```python
from build123d import *

# Parameters (mm, degrees)
SKETCH_R        = 16
PAD_DEPTH       = 35
SKETCH001_R     = 14
POCKET_DEPTH    = 23
SKETCH002_R     = 3.98
PAD001_DEPTH    = 10
SKETCH003_W     = 5.2
SKETCH003_H     = 1.2
POCKET001_DEPTH = 10
SKETCH004_W     = 4.2
SKETCH004_H     = 32.681076
POCKET002_DEPTH = 10


with BuildPart() as part:
    # Sketch → Pad (new body)
    with BuildSketch(Plane.XY):
        Circle(SKETCH_R)
    extrude(amount=PAD_DEPTH)

    # Sketch001 (on Face2 of Pad) → Pocket (cut)
    with BuildSketch(Plane(origin=(0, 0, 0), x_dir=(1, 0, 0), z_dir=(0, 0, -1))):
        Circle(SKETCH001_R)
    extrude(amount=-POCKET_DEPTH, mode=Mode.SUBTRACT)

    # Sketch002 (on Face5 of Pocket) → Pad001 (join)
    with BuildSketch(Plane(origin=(0, 0, 23), x_dir=(1, 0, 0), z_dir=(0, 0, -1))):
        Circle(SKETCH002_R)
    extrude(amount=PAD001_DEPTH)

    # Sketch003 (on Face3 of Pad001) → Pocket001 (cut)
    with BuildSketch(Plane.XY.offset(35)):
        Rectangle(SKETCH003_W, SKETCH003_H)
    extrude(amount=-POCKET001_DEPTH, mode=Mode.SUBTRACT)

    # Sketch004 (on Face3 of Pocket001) → Pocket002 (cut)
    with BuildSketch(Plane.XY.offset(35)):
        with Locations((0, -0.015375)):
            Rectangle(SKETCH004_W, SKETCH004_H)
    extrude(amount=-POCKET002_DEPTH, mode=Mode.SUBTRACT)


solid = part.part
```
Source: CAD feature listing. Evaluate the final solid. Frame: model axes, mm. A direction names the side the tool comes from. Round coordinates to 2 decimals unless told otherwise and drop trailing zeros. Loops run counter-clockwise (first coordinate to the right, second up) from the corner with the lowest first, then second, coordinate; pieces in that order, holes last. Notation, with made-up numbers: M -30,3 L 15,3 A33 cw 15,33 Z; hole C 13,43.5 d6. An arc over 180 degrees is marked long. Use a Markdown table: item, result. Add a question column.
1. Pull-direction query (X, two-part tool) for faces 1 (the flat face through (-8, 0, 35)), 2 (the flat face through (2.6, 0, 30)), 3 (the cylindrical face through (-3.47, -15.62, 17.26)), 4 (the cylindrical face through (12.932, 5.362, 11.339)); classes: +X half, -X half, draft (parallel to the pull), parting line (faces both ways), or undercut.
2. Contact query for flat-ended pins moving along their axis: pin 1 (3 mm diameter, centred on x = -7, z = 14.5, fed in from -Y) (3 decimals); pin 2 (4 mm diameter, centred on x = 4.5, y = -1.5, fed in from -Z); pin 3 (10 mm diameter, centred on y = -12, z = 23, fed in from -X). Output: stop coordinate, or through.
3. Set-up query: faces 5 (the flat face through (7, 0, 35)), 6 (the flat face through (-2.1, 8, 30)), 7 (the flat face through (-2.6, 0, 30)), 8 (the flat face through (3, 3, 23)). Return all of +Z, -Z, +X, -X, +Y, -Y with unobstructed straight access to the full face (end or side cutting, diameter ignored); none if empty.
4. Ray query, line 1 along Y through (x, z) = (0, 10.5); line 2 along Y through (x, z) = (0, 15); line 3 along X through (y, z) = (2, 26). Return the intervals inside material, ascending. Write a range as [from, to].
5. Cut plane A-A, the plane z = 27.5. Output: boundary loops of the cut face in (x, y), and give its area (3 significant figures).
6. Cut plane D-D, the plane x = 0. Output: boundary loops of the cut face in (y, z), and give its area (3 significant figures).
7. Cut plane C-C, the plane z = 16.5. Output: boundary loops of the cut face in (x, y).
8. Cut plane B-B, the plane y = 0. Output: boundary loops of the cut face in (x, z), and give its area (3 significant figures).
Solution:
| question | item | result |
|---|---|---|
| 1 | face 1 | draft |
| 1 | face 2 | undercut |
| 1 | face 3 | parting line |
| 1 | face 4 | undercut |
| 2 | pin 1 | stops at y = -15.025 |
| 2 | pin 2 | stops at z = 13 |
| 2 | pin 3 | stops at x = -14.39 |
| 3 | face 5 | +Z, +X, -X, +Y, -Y |
| 3 | face 6 | +Z, +Y, -Y |
| 3 | face 7 | +Z |
| 3 | face 8 | -Z |
| 4 | line 1 | y = [-16, -14], [14, 16] |
| 4 | line 2 | y = [-16, -14], [-3.98, 3.98], [14, 16] |
| 4 | line 3 | x = [-15.87, -2.1], [2.1, 15.87] |
| 5 | outline | M -2.6,-0.6 L -2.6,0.6 L -2.1,0.6 L -2.1,15.86 A16 ccw -2.1,-15.86 L -2.1,-0.6 Z; M 2.1,-15.86 A16 ccw 2.1,15.86 L 2.1,0.6 L 2.6,0.6 L 2.6,-0.6 L 2.1,-0.6 Z |
| 5 | area | 669 mm2 |
| 6 | outline | M -16,0 L -14,0 L -14,23 L -3.98,23 L -3.98,13 L 3.98,13 L 3.98,23 L 14,23 L 14,0 L 16,0 L 16,25 L -16,25 Z |
| 6 | area | 236 mm2 |
| 7 | outline | C 0,0 d32; C 0,0 d7.96; hole C 0,0 d28 |
| 8 | outline | M -16,0 L -14,0 L -14,23 L -3.98,23 L -3.98,13 L 3.98,13 L 3.98,23 L 14,23 L 14,0 L 16,0 L 16,35 L 2.6,35 L 2.6,25 L -2.6,25 L -2.6,35 L -16,35 Z |
| 8 | area | 504 mm2 |
